```python
from build123d import *

# Parameters (mm, degrees)
SKETCH5_R                = 154.617689271
BOSS_EXTRUDE4_DEPTH      = 3.175
BOSS_EXTRUDE9_DEPTH      = 95.25
CUT_EXTRUDE1_START       = -95.25
CUT_EXTRUDE1_DEPTH       = 82.55
BOSS_EXTRUDE10_DEPTH     = 12.7
CUT_EXTRUDE11_DEPTH      = 6.096
CUT_EXTRUDE11_DRAFT      = -10
FILLET2_R                = 25.4
CIRPATTERN7_COUNT        = 4
CIRPATTERN7_COPY_1_DEPTH = 6.096
CIRPATTERN7_COPY_1_DRAFT = -10
CIRPATTERN7_COPY_2_DEPTH = 6.096
CIRPATTERN7_COPY_2_DRAFT = -10
CIRPATTERN7_COPY_3_DEPTH = 6.096
CIRPATTERN7_COPY_3_DRAFT = -10
FILLET2_OF_CIRPATTERN7_R = 25.4
SKETCH26_R               = 154.617689271
CUT_EXTRUDE9_DEPTH       = 6.35
SKETCH27_R               = 2.249999945
CUT_EXTRUDE12_DEPTH      = 35.000000104
CIRPATTERN8_COUNT        = 4


# Read off the part's stored shape, not the designer's step: Cut-Extrude11
with BuildPart() as part:
    # Sketch5 → Boss-Extrude4 (new, symmetric)
    with BuildSketch(Plane(origin=(0, 0, 0), x_dir=(1, 0, 0), z_dir=(0, 1, 0))):
        with Locations(Location((0, 0, 0), (0, 0, 270))):
            Circle(SKETCH5_R)
    extrude(amount=BOSS_EXTRUDE4_DEPTH, both=True)

    # Sketch15 → Boss-Extrude9 (add)
    with BuildSketch(Plane(origin=(0, 3.175, 0), x_dir=(1, 0, 0), z_dir=(0, 1, 0))):
        Polygon((0, 8.980256121), (94.292689271, 103.272945392), (103.272945392, 94.292689271), (8.980256121, 0), (0, 0), align=None)
    boss_extrude9 = extrude(amount=BOSS_EXTRUDE9_DEPTH)

    # Sketch17 → Cut-Extrude1 (cut)
    with BuildSketch(Plane(origin=(0, 98.425, 0), x_dir=(1, 0, 0), z_dir=(0, 1, 0)).offset(CUT_EXTRUDE1_START)):
        Polygon((13.470384182, 4.490128061), (119.126854284, 110.146598163), (110.146598163, 119.126854284), (4.490128061, 13.470384182), align=None)
    cut_extrude1 = extrude(amount=CUT_EXTRUDE1_DEPTH, mode=Mode.SUBTRACT)

    # Sketch19 → Boss-Extrude10 (add)
    with BuildSketch(Plane(origin=(0, 98.425, 0), x_dir=(1, 0, 0), z_dir=(0, 1, 0))):
        Polygon((60.325, 106.992689271), (81.592689271, 106.992689271), (106.992689271, 106.992689271), (106.992689271, 81.592689271), (106.992689271, 60.325), (77.102561211, 60.325), (77.102561211, 77.102561211), (60.325, 77.102561211), align=None)
    boss_extrude10 = extrude(amount=-BOSS_EXTRUDE10_DEPTH)


with BuildPart() as cut_extrude11_tool:
    # Cut-Extrude11 outline → Cut-Extrude11 (with draft: the straight prism first)
    with BuildSketch(Plane(origin=(0, 92.329, 0), x_dir=(1, 0, 0), z_dir=(0, 1, 0))):
        Polygon((83.452561211, 60.325), (100.642689271, 60.325), (100.642689271, 100.642689271), (60.325, 100.642689271), (60.325, 83.452561211), (83.452561211, 83.452561211), align=None)
    extrude(amount=CUT_EXTRUDE11_DEPTH)
    # Cut-Extrude11: the draft: its side faces are tilted about the plane it starts from
    cut_extrude11_sides = [cut_extrude11_tool.faces().sort_by_distance(p)[0] for p in [
        (92.047625241, 95.377, -60.325),
        (100.642689271, 95.377, -80.483844636),
        (80.483844635, 95.377, -100.642689271),
        (60.325, 95.377, -92.047625241),
        (71.888780606, 95.377, -83.452561211),
        (83.452561211, 95.377, -71.888780606),
    ]]
    draft(cut_extrude11_sides, Plane(origin=(0, 92.329, 0), x_dir=(1, 0, 0), z_dir=(0, 1, 0)), CUT_EXTRUDE11_DRAFT)


with BuildPart() as part_1:
    add(part.part)

    # Cut-Extrude11: cut by cut_extrude11_tool
    add(cut_extrude11_tool.part, mode=Mode.SUBTRACT)

    # Fillet2
    fillet2_edges = [part_1.edges().sort_by_distance(p)[0] for p in [
        (8.980256121, 85.725, -8.980256121),
    ]]
    fillet(fillet2_edges, radius=FILLET2_R)

    # CirPattern7: Boss-Extrude9, Cut-Extrude1, Boss-Extrude10 ×4 about axis
    cirpattern7_axis = Axis((0, 0, 0), (0, 1, 0))
    add([boss_extrude9.rotate(cirpattern7_axis, i * 360 / CIRPATTERN7_COUNT) for i in range(1, CIRPATTERN7_COUNT)])
    add([cut_extrude1.rotate(cirpattern7_axis, i * 360 / CIRPATTERN7_COUNT) for i in range(1, CIRPATTERN7_COUNT)], mode=Mode.SUBTRACT)
    add([boss_extrude10.rotate(cirpattern7_axis, i * 360 / CIRPATTERN7_COUNT) for i in range(1, CIRPATTERN7_COUNT)])


with BuildPart() as cirpattern7_copy_1_tool:
    # CirPattern7 copy 1 sketch → CirPattern7 copy 1 (with draft: the straight prism first)
    with BuildSketch(Plane(origin=(0, 92.329, 0), x_dir=(0, 0, -1), z_dir=(0, 1, 0))):
        Polygon((83.452561211, 60.325), (100.642689271, 60.325), (100.642689271, 100.642689271), (60.325, 100.642689271), (60.325, 83.452561211), (83.452561211, 83.452561211), align=None)
    extrude(amount=CIRPATTERN7_COPY_1_DEPTH)
    # CirPattern7 copy 1: the draft: its side faces are tilted about the plane it starts from
    cirpattern7_copy_1_sides = [cirpattern7_copy_1_tool.faces().sort_by_distance(p)[0] for p in [
        (-60.325, 95.377, -92.047625241),
        (-80.483844636, 95.377, -100.642689271),
        (-100.642689271, 95.377, -80.483844635),
        (-92.047625241, 95.377, -60.325),
        (-83.452561211, 95.377, -71.888780606),
        (-71.888780606, 95.377, -83.452561211),
    ]]
    draft(cirpattern7_copy_1_sides, Plane(origin=(0, 92.329, 0), x_dir=(0, 0, -1), z_dir=(0, 1, 0)), CIRPATTERN7_COPY_1_DRAFT)


with BuildPart() as part_2:
    add(part_1.part)

    # CirPattern7 copy 1: cut by cirpattern7_copy_1_tool
    add(cirpattern7_copy_1_tool.part, mode=Mode.SUBTRACT)


with BuildPart() as cirpattern7_copy_2_tool:
    # CirPattern7 copy 2 sketch → CirPattern7 copy 2 (with draft: the straight prism first)
    with BuildSketch(Plane(origin=(0, 92.329, 0), x_dir=(-1, 0, 0), z_dir=(0, 1, 0))):
        Polygon((83.452561211, 60.325), (100.642689271, 60.325), (100.642689271, 100.642689271), (60.325, 100.642689271), (60.325, 83.452561211), (83.452561211, 83.452561211), align=None)
    extrude(amount=CIRPATTERN7_COPY_2_DEPTH)
    # CirPattern7 copy 2: the draft: its side faces are tilted about the plane it starts from
    cirpattern7_copy_2_sides = [cirpattern7_copy_2_tool.faces().sort_by_distance(p)[0] for p in [
        (-92.047625241, 95.377, 60.325),
        (-100.642689271, 95.377, 80.483844636),
        (-80.483844635, 95.377, 100.642689271),
        (-60.325, 95.377, 92.047625241),
        (-71.888780606, 95.377, 83.452561211),
        (-83.452561211, 95.377, 71.888780606),
    ]]
    draft(cirpattern7_copy_2_sides, Plane(origin=(0, 92.329, 0), x_dir=(-1, 0, 0), z_dir=(0, 1, 0)), CIRPATTERN7_COPY_2_DRAFT)


with BuildPart() as part_3:
    add(part_2.part)

    # CirPattern7 copy 2: cut by cirpattern7_copy_2_tool
    add(cirpattern7_copy_2_tool.part, mode=Mode.SUBTRACT)


with BuildPart() as cirpattern7_copy_3_tool:
    # CirPattern7 copy 3 sketch → CirPattern7 copy 3 (with draft: the straight prism first)
    with BuildSketch(Plane.ZX.offset(92.329)):
        Polygon((83.452561211, 60.325), (100.642689271, 60.325), (100.642689271, 100.642689271), (60.325, 100.642689271), (60.325, 83.452561211), (83.452561211, 83.452561211), align=None)
    extrude(amount=CIRPATTERN7_COPY_3_DEPTH)
    # CirPattern7 copy 3: the draft: its side faces are tilted about the plane it starts from
    cirpattern7_copy_3_sides = [cirpattern7_copy_3_tool.faces().sort_by_distance(p)[0] for p in [
        (60.325, 95.377, 92.047625241),
        (80.483844636, 95.377, 100.642689271),
        (100.642689271, 95.377, 80.483844635),
        (92.047625241, 95.377, 60.325),
        (83.452561211, 95.377, 71.888780606),
        (71.888780606, 95.377, 83.452561211),
    ]]
    draft(cirpattern7_copy_3_sides, Plane.ZX.offset(92.329), CIRPATTERN7_COPY_3_DRAFT)


with BuildPart() as part_4:
    add(part_3.part)

    # CirPattern7 copy 3: cut by cirpattern7_copy_3_tool
    add(cirpattern7_copy_3_tool.part, mode=Mode.SUBTRACT)

    # Fillet2 of CirPattern7
    fillet2_of_cirpattern7_edges = [part_4.edges().sort_by_distance(p)[0] for p in [
        (-8.980256121, 85.725, -8.980256121),
        (-8.980256121, 85.725, 8.980256121),
        (8.980256121, 85.725, 8.980256121),
    ]]
    fillet(fillet2_of_cirpattern7_edges, radius=FILLET2_OF_CIRPATTERN7_R)

    # Sketch26 → Cut-Extrude9 (cut)
    with BuildSketch(Plane(origin=(0, 3.175, 0), x_dir=(1, 0, 0), z_dir=(0, 1, 0))):
        Circle(SKETCH26_R)
    extrude(amount=-CUT_EXTRUDE9_DEPTH, mode=Mode.SUBTRACT)

    # Sketch27 → Cut-Extrude12 (cut)
    with BuildSketch(Plane.XZ.offset(-3.175)):
        with Locations(Location((5.388153673, 5.388153673, 0), (0, 0, 270))):
            Circle(SKETCH27_R)
    cut_extrude12 = extrude(amount=-CUT_EXTRUDE12_DEPTH, mode=Mode.SUBTRACT)

    # CirPattern8: Cut-Extrude12 ×4 about axis
    cirpattern8_axis = Axis((0, 0, 0), (0, 1, 0))
    for i in range(1, CIRPATTERN8_COUNT):
        add(cut_extrude12.rotate(cirpattern8_axis, i * 360 / CIRPATTERN8_COUNT), mode=Mode.SUBTRACT)


solid = part_4.part
```
Verification items for the finished model (mm, model axes). A direction names the side the tool comes from. Coordinates: 2 decimals unless noted, no trailing zeros. Loops run counter-clockwise (first coordinate to the right, second up) from the corner with the lowest first, then second, coordinate; pieces in that order, holes last. Notation, with made-up numbers: (26, 36) - (81, 36) arc R9 ccw to (81, 45) - close; hole circle Ø11 at (-29, 27). An arc over 180 degrees is marked (long way). Return JSON: item names as keys, results as strings.
1. Thickness scan on L1, parallel to X at y = 89, z = -79 (3 decimals); L2, parallel to X at y = 93, z = 22.5; L3, parallel to Z at x = -12.5, y = 11. Record the ranges inside material, lowest first.
Established:
{"L1": "x = -106.993 to -60.325, 60.325 to 106.993", "L2": "x = -31.48 to -13.52, 13.52 to 31.48", "L3": "z = -5.46 to -3.52, 3.52 to 5.46"}
2. Section check D-D, the plane z = 52.5. Record the boundary of the cut face in (x, y) (3 decimals), then the cut area to 3 significant figures.
Established:
{"outline": "(-61.48, 85.725) - (-43.52, 85.725) - (-43.52, 98.425) - (-61.48, 98.425) - close; (43.52, 85.725) - (61.48, 85.725) - (61.48, 98.425) - (43.52, 98.425) - close", "area": "456 mm2"}
3. Mould release check, pull along X, two halves, no side actions. Record for faces 4 (the flat face through (60.325, 91, 92)), 5 (the cylindrical face through (-14.165, 78.087, 14.039)), 6 (the flat face through (-64, 92, 77.103)), 7 (the flat face through (106.993, 92, -83)): +X half, -X half, draft (parallel to the pull), parting line (faces both ways), or undercut.
Established:
{"face 4": "undercut", "face 5": "-X half", "face 6": "undercut", "face 7": "+X half"}
4. Section check A-A, the plane z = -65.5. Record the boundary of the cut face in (x, y) (3 decimals).
Established:
{"outline": "(-106.993, 85.725) - (-77.103, 85.725) - (-77.103, 98.425) - (-82.378, 98.425) - (-83.453, 92.329) - (-100.643, 92.329) - (-101.718, 98.425) - (-106.993, 98.425) - close; (-74.48, 85.725) - (-56.52, 85.725) - (-56.52, 98.425) - (-74.48, 98.425) - close; (56.52, 85.725) - (74.48, 85.725) - (74.48, 98.425) - (56.52, 98.425) - close; (77.103, 85.725) - (106.993, 85.725) - (106.993, 98.425) - (101.718, 98.425) - (100.643, 92.329) - (83.453, 92.329) - (82.378, 98.425) - (77.103, 98.425) - close"}
5. Section check B-B, the plane x = -40. Record the boundary of the cut face in (y, z) (3 decimals).
Established:
{"outline": "(85.725, -48.98) - (98.425, -48.98) - (98.425, -31.02) - (85.725, -31.02) - close; (85.725, 31.02) - (98.425, 31.02) - (98.425, 48.98) - (85.725, 48.98) - close"}
6. Tool access check on faces 1 (the flat face through (-80.73, 95.33, -101.17)), 2 (the flat face through (-8.92, 31.35, 9.04)), 3 (the flat face through (84, 92, -106.993)). Record the directions out of +Z, -Z, +X, -X, +Y, -Y that give a thin tool (end or side, any length) a straight path to the whole face; none if there is none.
Established:
{"face 1": "+Y", "face 2": "+Z, -X, -Y", "face 3": "-Z, +X, -X, +Y, -Y"}
7. Go/stop test with flat-tipped pins: pin 1 (2 mm diameter, centred on x = -25, z = 24, fed in from -Y); pin 2 (12 mm diameter, centred on y = 53, z = 10, fed in from -X); pin 3 (12 mm diameter, centred on x = -90, z = -84.5, fed in from +Y). Record where each tip stops, or that it passes through.
Established:
{"pin 1": "stops at y = 85.33", "pin 2": "stops at x = -13.47", "pin 3": "stops at y = 92.33"}
